```python
from build123d import *

# Parameters (mm, degrees)
SKETCH1_R           = 6.5
SKETCH1_R_2         = 4.5
BOSS_EXTRUDE1_DEPTH = 4
FILLET1_R           = 10


with BuildPart() as part:
    # Sketch1 → Boss-Extrude1 (new body)
    # profile 1 of 3: a face of its own
    with BuildSketch(Plane.XY):
        with BuildLine():
            ThreePointArc((6.5, 0), (6.475721286, -0.561278744), (6.403066514, -1.118364526))
            Line((6.403066514, -1.118364526), (16, 4))
            Line((16, 4), (104, 4))
            Line((104, 4), (113.596933486, -1.118364526))
            ThreePointArc((113.596933486, -1.118364526), (114.264705882, 3.058823529), (117.361639368, 5.940459004))
            Line((117.361639368, 5.940459004), (106, 12))
            Line((106, 12), (14, 12))
            Line((14, 12), (2.638360632, 5.940459004))
            ThreePointArc((2.638360632, 5.940459004), (5.449740549, 3.542644203), (6.5, 0))
        make_face()
    # profile 2 of 3: a face of its own
    with BuildSketch(Plane.XY):
        Circle(SKETCH1_R)
        Circle(SKETCH1_R_2, mode=Mode.SUBTRACT)
    # profile 3 of 3: a face of its own
    with BuildSketch(Plane.XY):
        with Locations((120, 0)):
            Circle(SKETCH1_R)
        with Locations((120, 0)):
            Circle(SKETCH1_R_2, mode=Mode.SUBTRACT)
    extrude(amount=BOSS_EXTRUDE1_DEPTH)

    # Fillet1
    fillet1_edges = [part.edges().sort_by_distance(p)[0] for p in [
        (104, 4, 2),
        (16, 4, 2),
        (6.403066514, -1.118364526, 2),
        (2.638360632, 5.940459004, 2),
        (14, 12, 2),
        (106, 12, 2),
        (117.361639368, 5.940459004, 2),
        (113.596933486, -1.118364526, 2),
    ]]
    fillet(fillet1_edges, radius=FILLET1_R)


solid = part.part
```
Model file for the job. Use its own axes, mm. A direction names the side the tool comes from. Coordinates: 2 decimals unless noted, no trailing zeros. Write each loop counter-clockwise with the first axis right and the second up, starting at its lowest first coordinate (ties: lowest second). Pieces come first, ordered by that corner, then holes. Notation, with made-up numbers: (75, -15.75) - (120, -15.75) arc R24 cw to (120, 7.25) - close; hole circle Ø6 at (-40, -11). An arc over 180 degrees is marked (long way). Use a Markdown table: item, result. Add a question column.
Item 1: Band-saw the part on A-A, the plane y = -2. Write the cut outline in (x, z), and give its area (3 significant figures).
Item 2: Drill centre lines: line 1 along Y through (x, z) = (120, 1.25); line 2 along X through (y, z) = (1.5, 2.7); line 3 along X through (y, z) = (1.75, 2.45). Where is each one in solid material? Low to high.
Item 3: Two-plate mould, pull along Y, no slides. Class faces 3 (the face through (115.504, 0.198, 1.972)), 4 (the face through (103.89, 3.71, 2.03)), 5 (the face through (3.25, 6.692, 2.028)): pulls with the +Y half, pulls with the -Y half, needs draft (parallel to the pull), parting line crosses it, or undercut.
Item 4: 3-axis set-ups, long thin cutter, end or side, ignore diameter. For faces 1 (the face through (125.64, -3.23, 1.97)), 2 (the face through (16.041, 3.693, 2.028)): which of +Z, -Z, +X, -X, +Y, -Y reach the whole face in a straight line?
Item 5: Drop flat-ended pins along their axis: pin 1 (5.5 mm diameter, centred on x = 0, y = 0, fed in from +Z); pin 2 (1 mm diameter, centred on x = 86, z = 2.5, fed in from -Y). Give the stop position or say it passes through.
Item 6: Band-saw the part on B-B, the plane z = 1.65. Write the cut outline in (x, y), and give its area (3 significant figures).
Item 7: Band-saw the part on C-C, the plane x = 89. Write the cut outline in (y, z), and give its area (3 significant figures).
A:
| question | item | result |
|---|---|---|
| 1 | outline | (-6.18, 0) - (-4.03, 0) - (-4.03, 4) - (-6.18, 4) - close; (4.03, 0) - (6.48, 0) - (6.48, 4) - (4.03, 4) - close; (113.52, 0) - (115.97, 0) - (115.97, 4) - (113.52, 4) - close; (124.03, 0) - (126.18, 0) - (126.18, 4) - (124.03, 4) - close |
| 1 | area | 36.8 mm² |
| 2 | line 1 | y = -6.5 to -4.5, 4.5 to 6.5 |
| 2 | line 2 | x = -6.32 to -4.24, 4.24 to 11.31, 108.69 to 115.76, 124.24 to 126.32 |
| 2 | line 3 | x = -6.26 to -4.15, 4.15 to 11.78, 108.22 to 115.85, 124.15 to 126.26 |
| 3 | face 3 | undercut |
| 3 | face 4 | pulls with the -Y half |
| 3 | face 5 | pulls with the +Y half |
| 4 | face 1 | +Z, -Z |
| 4 | face 2 | +Z, -Z, -Y |
| 5 | pin 1 | passes through |
| 5 | pin 2 | stops at y = 4 |
| 6 | outline | (0.44, 6.49) arc R6.5 ccw (long way) to (5.63, -3.25) arc R10 cw to (9.59, 0.58) - (13.79, 2.82) arc R10 cw to (18.5, 4) - (101.5, 4) arc R10 cw to (106.21, 2.82) - (110.41, 0.58) arc R10 cw to (114.37, -3.25) arc R6.5 ccw (long way) to (119.56, 6.49) arc R10 cw to (114.18, 7.64) - (108.21, 10.82) arc R10 ccw to (103.5, 12) - (16.5, 12) arc R10 ccw to (11.79, 10.82) - (5.82, 7.64) arc R10 cw to start; hole circle Ø9 at (0, 0); hole circle Ø9 at (120, 0) |
| 6 | area | 1,040 mm² |
| 7 | outline | (4, 0) - (12, 0) - (12, 4) - (4, 4) - close |
| 7 | area | 32.0 mm² |
